Read the model definition and answer for the solid it produces. Units are mm, in the model's axes. Face numbers are marked on the shaded views. A direction names the side the tool comes from. Coordinates: 2 decimals unless noted, no trailing zeros. Loops run counter-clockwise (first coordinate to the right, second up) from the corner with the lowest first, then second, coordinate; pieces in that order, holes last. Notation, with made-up numbers: (30.25, 72.25) -> (61.25, 72.25) arc R7 cw to (61.25, 80.25) -> close; hole circle Ø3 at (89.25, 86). An arc over 180 degrees is marked (long way). Answer as CSV lines item,"result".
```python
from build123d import *

# Parameters (mm, degrees)
BOSS_EXTRUDE4_DEPTH      = 250
BOSS_EXTRUDE4_DEPTH_BACK = 250
FILLET1_R                = 10
FILLET2_R                = 10
FILLET3_R                = 10
CUT_EXTRUDE1_DEPTH       = 100


with BuildPart() as part:
    # Sketch5 → Boss-Extrude4 (new, two sides: drawn at the far end of the back side and taken through both)
    with BuildSketch(Plane.XY.offset(-BOSS_EXTRUDE4_DEPTH_BACK)):
        with BuildLine():
            Line((0, 0), (672.171335821, 0))
            ThreePointArc((672.171335821, 0), (695.015340994, 7.164783727), (709.67572834, 26.092428616))
            Line((709.67572834, 26.092428616), (818.005303321, 318.223584322))
            ThreePointArc((818.005303321, 318.223584322), (820.376071762, 335.288930001), (815.348837324, 351.768416645))
            Line((815.348837324, 351.768416645), (740.331547095, 484.892737084))
            Line((740.331547095, 484.892737084), (370.482259657, 1141.220563707))
            ThreePointArc((370.482259657, 1141.220563707), (334.053202103, 1161.55204086), (299.344064495, 1138.4063941))
            Line((299.344064495, 1138.4063941), (211.46075369, 948.827148814))
            ThreePointArc((211.46075369, 948.827148814), (208.038304344, 936.789455071), (208.503214572, 924.283333024))
            Line((208.503214572, 924.283333024), (263.147839607, 646.500885254))
            ThreePointArc((263.147839607, 646.500885254), (263.711539672, 642.658800356), (263.900031848, 638.780160797))
            Line((263.900031848, 638.780160797), (263.900031848, 166.522987154))
            ThreePointArc((263.900031848, 166.522987154), (258.258035835, 146.04061517), (242.923653745, 131.336316241))
            Line((242.923653745, 131.336316241), (0, 0))
        make_face()
    extrude(amount=BOSS_EXTRUDE4_DEPTH + BOSS_EXTRUDE4_DEPTH_BACK)

    # Fillet1
    fillet1_edges = [part.edges().sort_by_distance(p)[0] for p in [
        (121.461826872, 65.66815812, 250),
        (336.085667911, 0, 250),
        (695.015340994, 7.164783727, 250),
        (763.840515831, 172.158006469, 250),
        (820.376071762, 335.288930001, 250),
        (592.91554849, 746.494490176, 250),
        (334.053202103, 1161.55204086, 250),
        (255.402409092, 1043.616771457, 250),
        (208.038304344, 936.789455071, 250),
        (235.825527089, 785.392109139, 250),
        (263.711539672, 642.658800356, 250),
        (263.900031848, 402.651573975, 250),
        (258.258035835, 146.04061517, 250),
    ]]
    fillet(fillet1_edges, radius=FILLET1_R)

    # Fillet2
    fillet2_edges = [part.edges().sort_by_distance(p)[0] for p in [
        (695.015340994, 7.164783727, -250),
        (763.840515831, 172.158006469, -250),
        (820.376071762, 335.288930001, -250),
        (592.91554849, 746.494490176, -250),
        (334.053202103, 1161.55204086, -250),
        (255.402409092, 1043.616771457, -250),
        (208.038304344, 936.789455071, -250),
        (235.825527089, 785.392109139, -250),
        (263.711539672, 642.658800356, -250),
        (121.461826872, 65.66815812, -250),
        (263.900031848, 402.651573975, -250),
        (258.258035835, 146.04061517, -250),
        (336.085667911, 0, -250),
    ]]
    fillet(fillet2_edges, radius=FILLET2_R)

    # Fillet3
    # the kernel refuses this fillet: 10 mm, written as the material it takes off along each edge
    with BuildSketch(Plane(origin=(39.52279504, 10, 240), x_dir=(0, -1, 0), z_dir=(0, 0, 1))) as fillet3_piece_1_section:
        Polygon((0, 0), (FILLET3_R, 0), (FILLET3_R, -FILLET3_R * 3.95227950403), (-FILLET3_R * 0.879666772827, -FILLET3_R * 0.475590547408), align=None)
    fillet3_piece_1 = extrude(amount=FILLET3_R, mode=Mode.PRIVATE)
    fillet3_piece_1 = fillet3_piece_1 - Plane(origin=(39.52279504, 10, 240), x_dir=(0.9694500432790283, 0.24528883706008733, 0), z_dir=(0, 0, 1)) * Sphere(FILLET3_R, mode=Mode.PRIVATE)
    add(fillet3_piece_1, mode=Mode.SUBTRACT)
    with BuildSketch(Plane(origin=(39.52279504, 10, -240), x_dir=(0, -1, 0), z_dir=(0, 0, -1))) as fillet3_piece_2_section:
        Polygon((0, 0), (FILLET3_R, 0), (FILLET3_R, FILLET3_R * 3.95227950403), (-FILLET3_R * 0.879666772827, FILLET3_R * 0.475590547408), align=None)
    fillet3_piece_2 = extrude(amount=FILLET3_R, mode=Mode.PRIVATE)
    fillet3_piece_2 = fillet3_piece_2 - Plane(origin=(39.52279504, 10, -240), x_dir=(0.9694500432790283, 0.24528883706008733, 0), z_dir=(0, 0, -1)) * Sphere(FILLET3_R, mode=Mode.PRIVATE)
    add(fillet3_piece_2, mode=Mode.SUBTRACT)
    with BuildSketch(Plane(origin=(0, 0, -240), x_dir=(1, 0, 0), z_dir=(0, 0, 1))) as fillet3_piece_3:
        with BuildLine():
            CenterArc((FILLET3_R * 3.95227950403, FILLET3_R), FILLET3_R, 118.397807475, 151.602192525)
            Line((FILLET3_R * 3.47668895662, FILLET3_R * 1.87966677283), (0, 0))
            Line((0, 0), (FILLET3_R * 3.95227950403, 0))
        make_face()
    extrude(amount=480, mode=Mode.SUBTRACT)

    # Sketch11 → Cut-Extrude1 (cut)
    with BuildSketch(Plane(origin=(769.289421626, 433.504619004, 0), x_dir=(0, 0, -1), z_dir=(0.8711981630321445, 0.4909315234627098, 0))):
        Polygon((-144.211144, 752.50763293), (148.55197, 752.50763293), (148.55197, 677.02589093), (-34.726412, 677.02589093), (-34.726412, 620.83659693), (135.288398, 620.83659693), (135.288398, 548.73101093), (-34.726412, 548.73101093), (-34.726412, 479.03698093), (153.857396, 479.03698093), (153.857396, 398.97330493), (-144.211144, 398.97330493), align=None)
        with BuildLine():
            Line((-51.366168, 257.313168), (-144.211144, 273.952938))
            add(Edge.make_bspline(
                [(-144.211144, 273.952938), (-136.494162, 303.534714), (-121.703274, 326.20336), (-99.838466, 341.958862)],
                knots=[0, 0, 0, 0, 1, 1, 1, 1], degree=3))
            add(Edge.make_bspline(
                [(-99.838466, 341.958862), (-77.812896, 357.714378), (-46.703804, 365.592122), (-6.511176, 365.592122)],
                knots=[0, 0, 0, 0, 1, 1, 1, 1], degree=3))
            add(Edge.make_bspline(
                [(-6.511176, 365.592122), (39.62994, 365.592122), (72.989812, 356.9909), (93.568468, 339.788456)],
                knots=[0, 0, 0, 0, 1, 1, 1, 1], degree=3))
            add(Edge.make_bspline(
                [(93.568468, 339.788456), (114.147082, 322.585998), (124.436396, 300.962382), (124.436396, 274.91758)],
                knots=[0, 0, 0, 0, 1, 1, 1, 1], degree=3))
            add(Edge.make_bspline(
                [(124.436396, 274.91758), (124.436396, 259.644378), (120.25636, 245.818104), (111.896288, 233.438772)],
                knots=[0, 0, 0, 0, 1, 1, 1, 1], degree=3))
            add(Edge.make_bspline(
                [(111.896288, 233.438772), (103.536216, 221.05944), (90.915734, 210.207438), (74.034828, 200.882752)],
                knots=[0, 0, 0, 0, 1, 1, 1, 1], degree=3))
            add(Edge.make_bspline(
                [(74.034828, 200.882752), (87.700312, 197.506554), (98.150402, 193.567668), (105.38507, 189.066094)],
                knots=[0, 0, 0, 0, 1, 1, 1, 1], degree=3))
            add(Edge.make_bspline(
                [(105.38507, 189.066094), (117.121312, 181.831426), (126.204848, 172.26559), (132.635664, 160.368586)],
                knots=[0, 0, 0, 0, 1, 1, 1, 1], degree=3))
            add(Edge.make_bspline(
                [(132.635664, 160.368586), (139.22727, 148.632316), (142.52308, 134.564906), (142.52308, 118.166328)],
                knots=[0, 0, 0, 0, 1, 1, 1, 1], degree=3))
            add(Edge.make_bspline(
                [(142.52308, 118.166328), (142.52308, 97.587686), (137.137266, 77.812896), (126.365638, 58.841986)],
                knots=[0, 0, 0, 0, 1, 1, 1, 1], degree=3))
            add(Edge.make_bspline(
                [(126.365638, 58.841986), (115.59401, 40.031838), (100.079658, 25.4821), (79.822582, 15.192814)],
                knots=[0, 0, 0, 0, 1, 1, 1, 1], degree=3))
            add(Edge.make_bspline(
                [(79.822582, 15.192814), (59.565478, 5.064276), (32.957946, 0), (0, 0)],
                knots=[0, 0, 0, 0, 1, 1, 1, 1], degree=3))
            add(Edge.make_bspline(
                [(0, 0), (-32.154108, 0), (-57.555834, 3.778096), (-76.205206, 11.334288)],
                knots=[0, 0, 0, 0, 1, 1, 1, 1], degree=3))
            add(Edge.make_bspline(
                [(-76.205206, 11.334288), (-94.693816, 18.890508), (-109.967018, 29.9033), (-122.024798, 44.372636)],
                knots=[0, 0, 0, 0, 1, 1, 1, 1], degree=3))
            add(Edge.make_bspline(
                [(-122.024798, 44.372636), (-133.92183, 59.002776), (-143.085754, 77.33061), (-149.51657, 99.356152)],
                knots=[0, 0, 0, 0, 1, 1, 1, 1], degree=3))
            Line((-149.51657, 99.356152), (-51.366168, 112.378574))
            add(Edge.make_bspline(
                [(-51.366168, 112.378574), (-47.50767, 92.603812), (-41.559154, 78.85794), (-33.520634, 71.140958)],
                knots=[0, 0, 0, 0, 1, 1, 1, 1], degree=3))
            add(Edge.make_bspline(
                [(-33.520634, 71.140958), (-25.321338, 63.584738), (-14.95165, 59.806628), (-2.411556, 59.806628)],
                knots=[0, 0, 0, 0, 1, 1, 1, 1], degree=3))
            add(Edge.make_bspline(
                [(-2.411556, 59.806628), (10.771628, 59.806628), (21.704032, 64.62974), (30.385642, 74.275978)],
                knots=[0, 0, 0, 0, 1, 1, 1, 1], degree=3))
            add(Edge.make_bspline(
                [(30.385642, 74.275978), (39.228028, 83.922202), (43.649214, 96.783848), (43.649214, 112.860888)],
                knots=[0, 0, 0, 0, 1, 1, 1, 1], degree=3))
            add(Edge.make_bspline(
                [(43.649214, 112.860888), (43.649214, 129.259494), (39.388804, 141.960364), (30.86797, 150.963498)],
                knots=[0, 0, 0, 0, 1, 1, 1, 1], degree=3))
            add(Edge.make_bspline(
                [(30.86797, 150.963498), (22.507898, 159.966632), (11.09318, 164.468206), (-3.376156, 164.468206)],
                knots=[0, 0, 0, 0, 1, 1, 1, 1], degree=3))
            add(Edge.make_bspline(
                [(-3.376156, 164.468206), (-11.093138, 164.468206), (-21.70399, 162.538964), (-35.208726, 158.680494)],
                knots=[0, 0, 0, 0, 1, 1, 1, 1], degree=3))
            Line((-35.208726, 158.680494), (-30.144478, 228.856796))
            add(Edge.make_bspline(
                [(-30.144478, 228.856796), (-24.678262, 228.052944), (-20.417838, 227.651018), (-17.363192, 227.651018)],
                knots=[0, 0, 0, 0, 1, 1, 1, 1], degree=3))
            add(Edge.make_bspline(
                [(-17.363192, 227.651018), (-4.501546, 227.651018), (6.189694, 231.75068), (14.710528, 239.94999)],
                knots=[0, 0, 0, 0, 1, 1, 1, 1], degree=3))
            add(Edge.make_bspline(
                [(14.710528, 239.94999), (23.39211, 248.149272), (27.732908, 257.875884), (27.732908, 269.129826)],
                knots=[0, 0, 0, 0, 1, 1, 1, 1], degree=3))
            add(Edge.make_bspline(
                [(27.732908, 269.129826), (27.732908, 279.901454), (24.5175, 288.502676), (18.086684, 294.933492)],
                knots=[0, 0, 0, 0, 1, 1, 1, 1], degree=3))
            add(Edge.make_bspline(
                [(18.086684, 294.933492), (11.655854, 301.364308), (2.813482, 304.57973), (-8.44046, 304.57973)],
                knots=[0, 0, 0, 0, 1, 1, 1, 1], degree=3))
            add(Edge.make_bspline(
                [(-8.44046, 304.57973), (-20.015912, 304.57973), (-29.420972, 301.04277), (-36.655654, 293.96885)],
                knots=[0, 0, 0, 0, 1, 1, 1, 1], degree=3))
            add(Edge.make_bspline(
                [(-36.655654, 293.96885), (-43.890322, 287.055734), (-48.793836, 274.837164), (-51.366168, 257.313168)],
                knots=[0, 0, 0, 0, 1, 1, 1, 1], degree=3))
        make_face()
    extrude(amount=-CUT_EXTRUDE1_DEPTH, mode=Mode.SUBTRACT)


solid = part.part
```
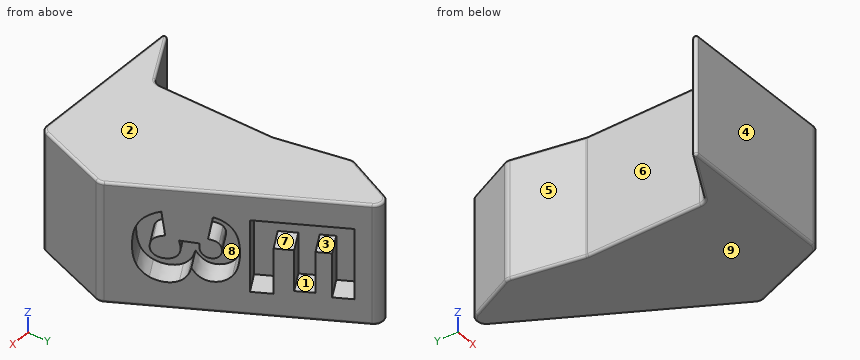
Q1. A cutting plane is placed at A-A, the plane z = 170. Write down the section's boundary in (x, y).
Results:
outline,"(34.77, 18.8) arc R10 ccw to (39.52, 0) -> (672.17, 0) arc R40 ccw to (709.68, 26.09) -> (818.01, 318.22) arc R40 ccw to (815.35, 351.77) -> (370.48, 1141.22) arc R40 ccw to (299.34, 1138.41) -> (211.46, 948.83) arc R40 ccw to (208.5, 924.28) -> (263.15, 646.5) arc R40 cw to (263.9, 638.78) -> (263.9, 166.52) arc R40 cw to (242.92, 131.34) -> close"
Q2. Find the intervals of material crossed by probe 1 along X at (y, z) = (274, -96); probe 2 along X at (y, z) = (902.5, -106.5); probe 3 along X at (y, z) = (337, -155), in increasing order. Write a range as [from, to].
Results:
probe 1,"x = [263.9, 801.61]"
probe 2,"x = [212.79, 390.22], [483.83, 505]"
probe 3,"x = [263.9, 820.2]"
Q3. For a pull along Z with two mould halves and no side action, classify the marked faces 6, 7, 8 and 9 as pulls with the +Z half, pulls with the -Z half, needs draft (parallel to the pull), parting line crosses it, or undercut.
Results:
face 6,"needs draft"
face 7,"undercut"
face 8,"undercut"
face 9,"pulls with the -Z half"
Q4. For the marked faces 1, 2, 3, 4 and 5, determine the directions among +Z, -Z, +X, -X, +Y, -Y from which every point of the face is accessible in a straight line to the end or side of a thin tool.
Results:
face 1,"none"
face 2,"+Z, +X, -X, +Y, -Y"
face 3,"+X"
face 4,"+Z, -Z, +X, -X, -Y"
face 5,"+Z, -Z, -X"
Q5. Given pin 1 Ø2 at (x, z) = (311.5, -7.5) entering from +Y; pin 2 Ø4 at (y, z) = (669.5, -53) entering from +X; pin 3 Ø4 at (y, z) = (357.5, -45.5) entering from -X, each flat-ended and moving along its own axis, determine where each tip first touches the part or whether it passes through.
Results:
pin 1,"stops at y = 1154.21"
pin 2,"stops at x = 522.65"
pin 3,"stops at x = 263.9"
